from build123d import *

# Parameters (mm, degrees)
EXTRUDE1_DEPTH           = 3.3
SKETCH11_W               = 3.5
SKETCH11_H               = 0.416666667
POINT_CUT_EXTRUDE8_DEPTH = 18.067754197
SKETCH16_R               = 3.112
CUT_EXTRUDE1_DEPTH       = 0.66


with BuildPart() as part:
    # Sketch1 → base-Revolve (revolve)
    with BuildSketch(Plane.XY, mode=Mode.PRIVATE) as base_revolve_sk:
        with BuildLine():
            Line((16, 2.5), (16, 0))
            Line((16, 0), (0, 0))
            Line((0, 0), (-2.64, 0))
            Line((-2.64, 0), (-3.3, 0))
            Line((-3.3, 0), (-3.3, 3.89))
            Line((-3.3, 3.89), (0, 3.89))
            Line((0, 3.89), (0, 2.2))
            ThreePointArc((0, 2.2), (0.058578644, 2.058578644), (0.2, 2))
            Line((0.2, 2), (0.5, 2))
            Line((0.5, 2), (1, 2.5))
            Line((1, 2.5), (16, 2.5))
        make_face()
    revolve(base_revolve_sk.sketch.rotate(Axis((0, 0, 0), (1, 0, 0)), 90), axis=Axis((0, 0, 0), (1, 0, 0)))

    # Sketch15 → Extrude1 (add)
    with BuildSketch(Plane.ZY.offset(3.3)):
        Polygon((-2.245892547, 3.89), (-4.491785094, 0), (-2.245892547, -3.89), (2.245892547, -3.89), (4.491785094, 0), (2.245892547, 3.89), align=None)
    extrude(amount=-EXTRUDE1_DEPTH)

    # Sketch8 → point_Cut-Revolve1 (revolve, cut)
    with BuildSketch(Plane.XY, mode=Mode.PRIVATE) as point_cut_revolve1_sk:
        Polygon((16, 0), (16.508, 0), (16.508, 3.008), (15.082013072, 3.008), (15.082013072, 2.5), (16, 1.97), align=None)
    revolve(point_cut_revolve1_sk.sketch.rotate(Axis((0, 0, 0), (1, 0, 0)), 90), axis=Axis((0, 0, 0), (1, 0, 0)), mode=Mode.SUBTRACT)

    # Sketch11 → point_Cut-Extrude8 (cut, through all)
    with BuildSketch(Plane.XY):
        with Locations((14.25, -0.208333334)):
            Rectangle(SKETCH11_W, SKETCH11_H)
    extrude(amount=POINT_CUT_EXTRUDE8_DEPTH, mode=Mode.SUBTRACT)

    # Sketch16 → Cut-Extrude1 (cut)
    with BuildSketch(Plane.ZY.offset(3.3)):
        Circle(SKETCH16_R)
    extrude(amount=-CUT_EXTRUDE1_DEPTH, mode=Mode.SUBTRACT)


solid = part.part
Input: part model. Units: mm. Frame: model coordinates. A direction names the side the tool comes from. Give positions to 0.01 mm unless a question says otherwise; leave off trailing zeros. Write each loop counter-clockwise with the first axis right and the second up, starting at its lowest first coordinate (ties: lowest second). Pieces come first, ordered by that corner, then holes. Notation, with made-up numbers: M -16,16 L 27,16 A23 ccw 27,52 Z; hole C 66,38.5 d7. An arc over 180 degrees is marked long. Use one line per item in the form item = value.
1. Reachability of faces 4 (the face through (-2.64, 0, 0)), 5 (the face through (-1.673, -1.918, -3.385)), 6 (the face through (14, 0, 1)) from +Z, -Z, +X, -X, +Y, -Y: full face, straight path, thin tool, end or side. Return the list, or none.
Outcome:
face_4 = -X
face_5 = -Z, +X, -X, -Y
face_6 = +Z, +X
2. Cut plane B-B on x = 8.25. Return loops of the section in (y, z), and give its area (3 significant figures).
Outcome:
outline = C 0,0 d5
area = 19.6 mm²
3. Ray query, L1, parallel to Y at x = -3.1, z = 0; L2, parallel to X at y = 1.5, z = -2.25; L3, parallel to X at y = 3, z = 1.75. Return the intervals inside material, ascending.
Outcome:
L1 = -3.89 to -3.11, 3.11 to 3.89
L2 = -2.64 to 0
L3 = -3.3 to 0
4. Cut plane A-A on x = -0.25. Return loops of the section in (y, z), and give its area (3 significant figures).
Outcome:
outline = M -3.89,-2.25 L 0,-4.49 L 3.89,-2.25 L 3.89,2.25 L 0,4.49 L -3.89,2.25 Z
area = 52.4 mm²
5. Mould query, pull axis Y, two halves, no side actions, for faces 1 (the face through (-1.673, 1.972, -3.353)), 2 (the face through (-2.975, 2.103, -2.294)), 3 (the face through (8.1, -0.1, -2.5)). Classes: released by +Y, released by -Y, zero draft, split by the parting line, or undercut.
Outcome:
face_1 = released by +Y
face_2 = undercut
face_3 = split by the parting line
6. First-contact query: P1, Ø1, axis at x = 11, y = -1.5, coming from the +Z side; P2, Ø1.2, axis at x = 14.5, z = 1, coming from the +Y side; P3, Ø0.5, axis at x = 15, y = 0, coming from the +Z side. Flat tips, straight axial feed; report the tip coordinate or a pass-through.
Outcome:
P1 = 2.29
P2 = 2.47
P3 = 2.5
